Can you work these out from the drawing? Everything is in mm from the part's minimum corner. Round coordinates to 2 decimals unless told otherwise and drop trailing zeros. Write each loop counter-clockwise with the first axis right and the second up, starting at its lowest first coordinate (ties: lowest second). Pieces come first, ordered by that corner, then holes. Notation, with made-up numbers: (47.25, 88) -> (67.25, 88) arc R30 ccw to (67.25, 114) -> close; hole circle Ø7 at (-26, -35). An arc over 180 degrees is marked (long way). Answer as CSV lines item,"result".
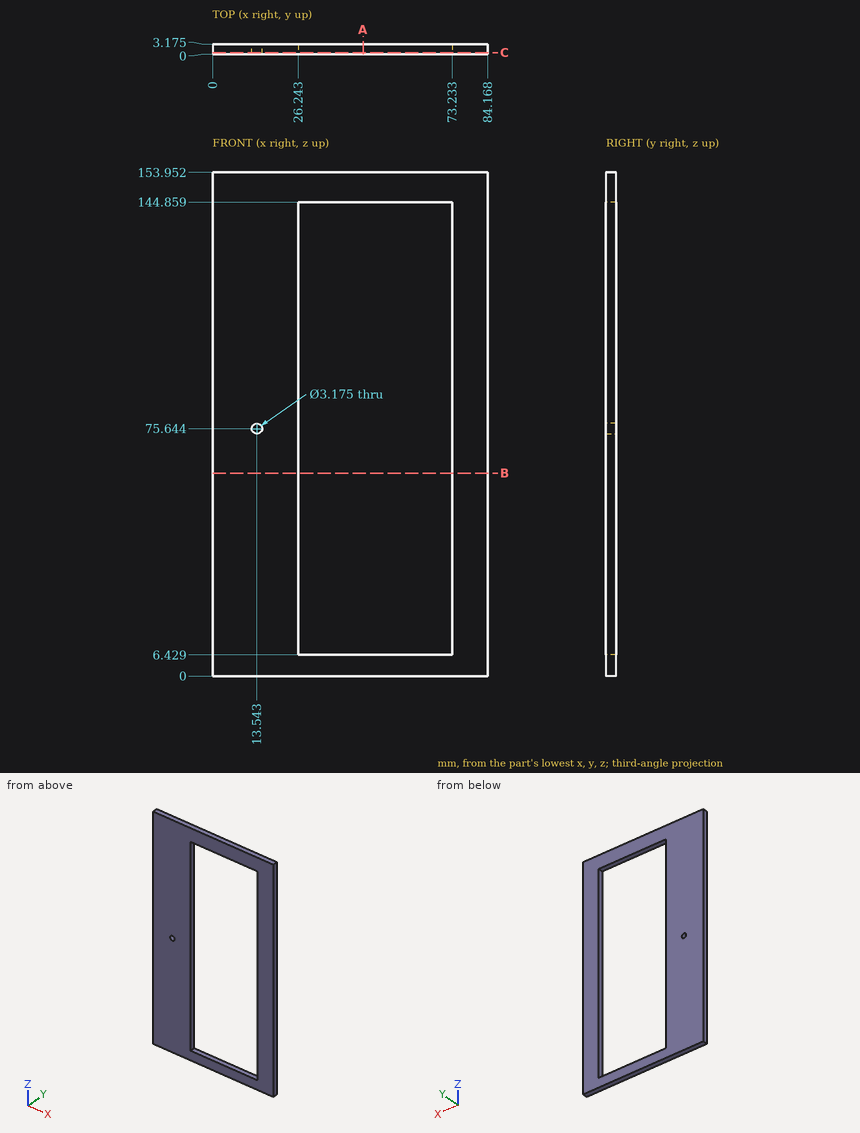
Item 1: Suppose I cut it at C-C, the plane y = 0.5. List the corners of the cut face in (x, z) for me (1 decimal).
Results found:
outline,"(0, 0) -> (84.2, 0) -> (84.2, 154) -> (0, 154) -> close; hole circle Ø3.2 at (13.5, 75.6); hole (26.2, 6.4) -> (73.2, 6.4) -> (73.2, 144.9) -> (26.2, 144.9) -> close"
Item 2: Will this pin go through, and if not, where does the flat tip stop? pin 1 (1.6 mm diameter, centred on x = 41.5, y = 2, fed in from -Z).
Results found:
pin 1,"stops at z = 0"
Item 3: I need wall thicknesses on L1, parallel to Z at x = 32.5, y = 0.65; L2, parallel to X at y = 0.3, z = 136.5. Which ranges of each line are inside material? Lowest first, please.
Results found:
L1,"z = 0 to 6.43, 144.86 to 153.95"
L2,"x = 0 to 26.24, 73.23 to 84.17"
Item 4: Suppose I cut it at B-B, the plane z = 62. List the corners of the cut face in (x, y) for me (1 decimal).
Results found:
outline,"(0, 0) -> (26.2, 0) -> (26.2, 3.2) -> (0, 3.2) -> close; (73.2, 0) -> (84.2, 0) -> (84.2, 3.2) -> (73.2, 3.2) -> close"
Item 5: Suppose I cut it at A-A, the plane x = 46. List the corners of the cut face in (y, z) for me (1 decimal).
Results found:
outline,"(0, 0) -> (3.2, 0) -> (3.2, 6.4) -> (0, 6.4) -> close; (0, 144.9) -> (3.2, 144.9) -> (3.2, 154) -> (0, 154) -> close"
